from build123d import *

# Parameters (mm, degrees)
SKETCH020_R  = 1.5
PAD005_DEPTH = 5
SKETCH021_R  = 1.5
PAD007_DEPTH = 5
SKETCH018_R  = 1.5
PAD004_DEPTH = 5
SKETCH017_R  = 1.5
PAD008_DEPTH = 5
SKETCH025_W  = 25
SKETCH025_H  = 10
SKETCH025_R  = 1.25
PAD014_DEPTH = 5
FILLET_R     = 0.5


with BuildPart() as body012:
    # Sketch020 → Pad005 (new body)
    with BuildSketch(Plane(origin=(0.02, 0, 0), x_dir=(1, 0, 0), z_dir=(0, -1, 0))):
        Polygon((0.683099, -4), (2.5, -4), (2.5, 4), (0.683099, 4), (-2.5, 0.816901), (-2.5, -0.816901), align=None)
        Circle(SKETCH020_R, mode=Mode.SUBTRACT)
    extrude(amount=PAD005_DEPTH)


with BuildPart() as body012_1:
    # Body012 placement: moved
    add(body012.part.moved(Location((337.5, 453, 4.5))))


with BuildPart() as body013:
    # Sketch021 → Pad007 (new body)
    with BuildSketch(Plane(origin=(0.02, 0, 0), x_dir=(1, 0, 0), z_dir=(0, -1, 0))):
        Polygon((0.683099, -4), (2.5, -4), (2.5, 4), (0.683099, 4), (-2.5, 0.816901), (-2.5, -0.816901), align=None)
        Circle(SKETCH021_R, mode=Mode.SUBTRACT)
    extrude(amount=PAD007_DEPTH)


with BuildPart() as body013_1:
    # Body013 placement: moved
    add(body013.part.moved(Location((337.5, 443, 4.5))))


with BuildPart() as body010:
    # Sketch018 → Pad004 (new body)
    with BuildSketch(Plane(origin=(0.02, 0, 0), x_dir=(1, 0, 0), z_dir=(0, -1, 0))):
        Polygon((0.683099, -4), (2.5, -4), (2.5, 4), (0.683099, 4), (-2.5, 0.816901), (-2.5, -0.816901), align=None)
        Circle(SKETCH018_R, mode=Mode.SUBTRACT)
    extrude(amount=PAD004_DEPTH)


with BuildPart() as body010_1:
    # Body010 placement: moved
    add(body010.part.moved(Location((337.5, 297, 4.5))))


with BuildPart() as body009:
    # Sketch017 → Pad008 (new body)
    with BuildSketch(Plane(origin=(0.02, 0, 0), x_dir=(1, 0, 0), z_dir=(0, -1, 0))):
        Polygon((0.683099, -4), (2.5, -4), (2.5, 4), (0.683099, 4), (-2.5, 0.816901), (-2.5, -0.816901), align=None)
        Circle(SKETCH017_R, mode=Mode.SUBTRACT)
    extrude(amount=PAD008_DEPTH)


with BuildPart() as body009_1:
    # Body009 placement: moved
    add(body009.part.moved(Location((337.5, 307, 4.5))))


with BuildPart() as hinge_aileron:
    # Sketch025 → Pad014 (new body)
    with BuildSketch(Plane.YZ):
        Rectangle(SKETCH025_W, SKETCH025_H)
        with Locations((0, 2.498994)):
            Circle(SKETCH025_R, mode=Mode.SUBTRACT)
    extrude(amount=PAD014_DEPTH)

    # Fillet
    fillet_edges = [hinge_aileron.edges().sort_by_distance(p)[0] for p in [
        (2.5, 12.5, 5),
        (2.5, -12.5, 5),
        (0, 0, 5),
        (5, 0, 5),
    ]]
    fillet(fillet_edges, radius=FILLET_R)


with BuildPart() as hinge_aileron_1:
    # Body017 placement: moved
    add(hinge_aileron.part.moved(Location((375, 375, 5))))


with BuildPart() as aileron:
    # Sketch012 → AdditiveLoft001 section 0
    with BuildSketch(Plane(origin=(10, 498, 0), x_dir=(1, 0, 0), z_dir=(0, -1, 0))):
        Polygon((334.392927, 10.526054), (342, 8.93095), (349.6, 7.263928), (357.2, 5.557082), (364.8, 3.808816), (368.6, 2.920984), (372.4, 2.02673), (376.2, 1.12822), (380, 0), (376.2, -0.367308), (372.4, -0.506882), (368.6, -0.646418), (364.8, -0.785954), (357.2, -1.065064), (349.6, -1.344174), (342, -1.623284), (334.4, -1.902394), (330.0157, -2.063407), (330.0157, 11.43475), align=None)
    # Sketch014 → AdditiveLoft001 section 1
    with BuildSketch(Plane(origin=(10, 252, 0), x_dir=(1, 0, 0), z_dir=(0, -1, 0))):
        Polygon((334.392927, 10.526054), (342, 8.93095), (349.6, 7.263928), (357.2, 5.557082), (364.8, 3.808816), (368.6, 2.920984), (372.4, 2.02673), (376.2, 1.12822), (380, 0), (376.2, -0.367308), (372.4, -0.506882), (368.6, -0.646418), (364.8, -0.785954), (357.2, -1.065064), (349.6, -1.344174), (342, -1.623284), (334.4, -1.902394), (330.0157, -2.063407), (330.0157, 11.43475), align=None)
    loft()

    # Boolean002: union Body012, Body013, Body010, Body009
    add(body012_1.part)
    add(body013_1.part)
    add(body010_1.part)
    add(body009_1.part)

    # Boolean004: union hinge_aileron
    add(hinge_aileron_1.part)


solid = aileron.part
Geometry check sheet. Reference: the model listing, model coordinates, mm. A direction names the side the tool comes from. Coordinates: 2 decimals unless noted, no trailing zeros. Order: outer loops, then holes, each group sorted by start corner. A loop starts at its lowest first (then second) coordinate and runs counter-clockwise, first axis right, second up. Notation, with made-up numbers: (87, 50) - (125, 50) arc R22 ccw to (125, 86) - close; hole circle Ø7 at (69, 77). An arc over 180 degrees is marked (long way). One line per item, written item: value.
(1) Sectioned sample at B-B (x = 364). Enter the section's corners in (y, z), and give its area (3 significant figures).
Data:
outline: (252, -1.18) - (498, -1.18) - (498, 6.28) - (252, 6.28) - close
area: 1,830 mm^2
(2) Access from +Z, -Z, +X, -X, +Y, -Y to the whole of each face (thin tool, end or side, straight path). Record for faces 1 (the face through (339.1, 297, 5.4)), 2 (the face through (377, 375, 10)), 3 (the face through (339.1, 292, 5.4)), 4 (the face through (339.1, 453, 5.4)).
Data:
face 1: +Z, -Z, -X
face 2: +Z, +X, +Y, -Y
face 3: +Z, -Z, -X, -Y
face 4: +Z, -Z, -X, +Y
(3) Thickness scan on probe 1 along Y at (x, z) = (339.5, 5); probe 2 along Z at (x, y) = (337.52, 295.5); probe 3 along Z at (x, y) = (348, 338.5). Record the ranges inside material, lowest first. Write a range as from..to.
Data:
probe 1: y = 292..297, 302..307, 438..443, 448..453
probe 2: z = 1.18..3, 6..7.82
probe 3: z = -1.77..9.77
(4) Depth check by flat-ended pin: pin 1 Ø2.5 at (x, z) = (377.5, 7.5) entering from -Y; pin 2 Ø1.5 at (x, y) = (339, 305) entering from -Z; pin 3 Ø12 at (x, y) = (367.5, 320.5) entering from +Z. Enter the tip coordinate at first touch or a pass-through.
Data:
pin 1: stops at y = 362.5
pin 2: stops at z = 0.5
pin 3: stops at z = 6.84
(5) Sectioned sample at A-A (y = 475). Enter the section's corners in (x, z), and give its area (3 significant figures).
Data:
outline: (340.02, -2.06) - (374.8, -0.79) - (382.4, -0.51) - (386.2, -0.37) - (390, 0) - (386.2, 1.13) - (382.4, 2.03) - (378.6, 2.92) - (374.8, 3.81) - (367.2, 5.56) - (359.6, 7.26) - (352, 8.93) - (344.39, 10.53) - (340.02, 11.43) - close
area: 355 mm^2
(6) Sectioned sample at C-C (y = 371.5). Enter the section's corners in (x, z).
Data:
outline: (340.02, -2.06) - (374.8, -0.79) - (382.4, -0.51) - (386.2, -0.37) - (390, 0) - (386.2, 1.13) - (382.4, 2.03) - (380, 2.59) - (380, 9.5) arc R0.5 ccw to (379.5, 10) - (375.5, 10) arc R0.5 ccw to (375, 9.5) - (375, 3.76) - (374.8, 3.81) - (367.2, 5.56) - (359.6, 7.26) - (352, 8.93) - (344.39, 10.53) - (340.02, 11.43) - close
